For this review, use the dimensioned drawing (mm, ordinates from the lowest corner) and the shaded views. A direction names the side the tool comes from. Give positions to 0.01 mm unless a question says otherwise; leave off trailing zeros. Order: outer loops, then holes, each group sorted by start corner. A loop starts at its lowest first (then second) coordinate and runs counter-clockwise, first axis right, second up.
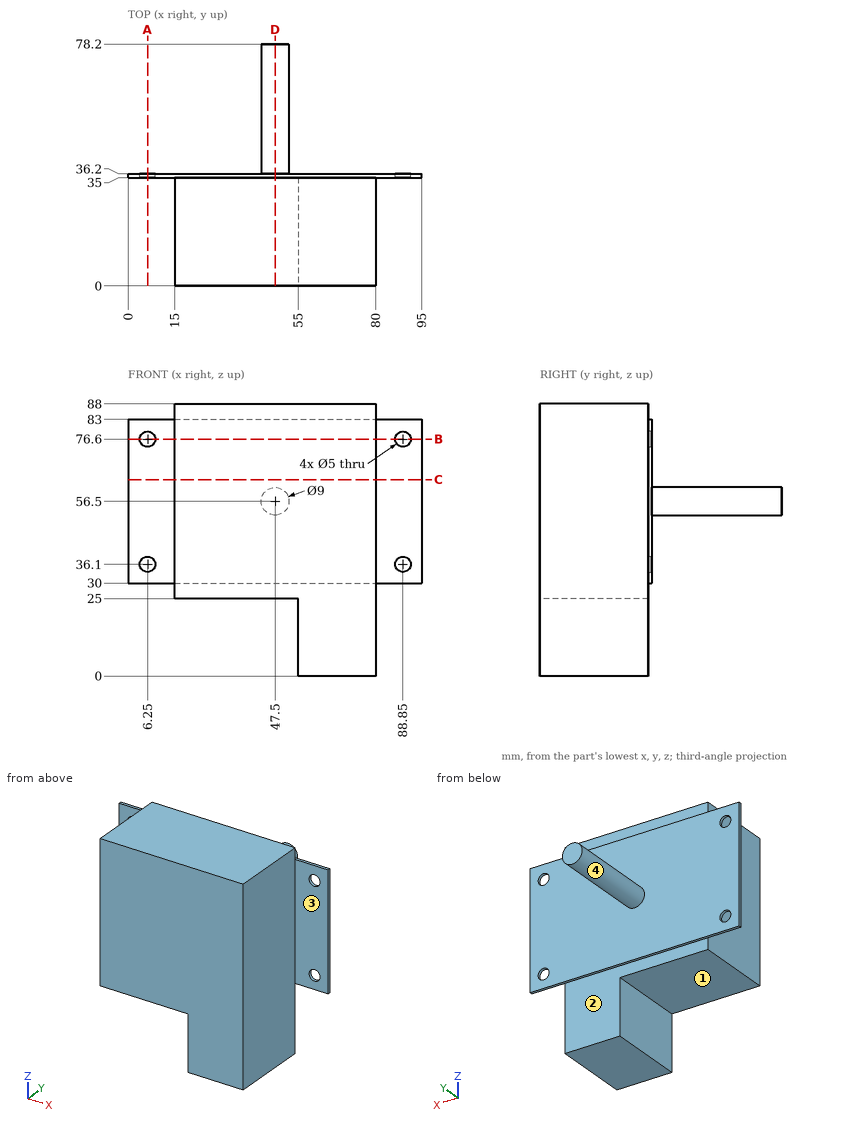
1. For pin 1 (7.5 mm diameter, centred on y = 22.5, z = 18, fed in from -X); pin 2 (10.5 mm diameter, centred on y = 17.5, z = 41, fed in from -X); pin 3 (17.5 mm diameter, centred on y = 25, z = 63, fed in from +X), all flat-tipped, find the tip position at first contact; note any pin that passes through.
Recorded:
pin 1: stops at x = 55
pin 2: stops at x = 15
pin 3: stops at x = 80
2. Take a section at C-C (z = 63.5). State the section outline as (x, y) points, then the cut area to 3 significant figures.
Recorded:
outline: (0, 35) - (15, 35) - (15, 0) - (80, 0) - (80, 35) - (95, 35) - (95, 36.2) - (0, 36.2) - close
area: 2,390 mm2
3. Take a section at A-A (x = 6.25). State the section outline as (y, z) points, then the cut area to 3 significant figures.
Recorded:
outline: (35, 30) - (36.2, 30) - (36.2, 33.6) - (35, 33.6) - close; (35, 38.6) - (36.2, 38.6) - (36.2, 74.1) - (35, 74.1) - close; (35, 79.1) - (36.2, 79.1) - (36.2, 83) - (35, 83) - close
area: 51.6 mm2
4. For line 1 along X through (y, z) = (35.85, 76.6); line 2 along Y through (x, z) = (62.5, 66.5); line 3 along Z through (x, y) = (73, 35.5), list the stretches that pass through material, from the lowest coordinate up.
Recorded:
line 1: x = 0 to 3.75, 8.75 to 86.35, 91.35 to 95
line 2: y = 0 to 36.2
line 3: z = 30 to 83
5. Machinability: for the marked faces 1, 2, 3 and 4, which of the approach directions +Z, -Z, +X, -X, +Y, -Y give a long, thin tool a straight path to every point of the face, cutting with its end or side? Answer none if there is none.
Recorded:
face 1: -Z, -X, +Y, -Y
face 2: -Z, +X, -X, +Y
face 3: +Z, -Z, +X, -Y
face 4: +Y
6. Take a section at D-D (x = 47.5). State the section outline as (y, z) points.
Recorded:
outline: (0, 25) - (35, 25) - (35, 30) - (36.2, 30) - (36.2, 52) - (78.2, 52) - (78.2, 61) - (36.2, 61) - (36.2, 83) - (35, 83) - (35, 88) - (0, 88) - close
7. Take a section at B-B (z = 76.6). State the section outline as (x, y) points, then the cut area to 3 significant figures.
Recorded:
outline: (0, 35) - (3.75, 35) - (3.75, 36.2) - (0, 36.2) - close; (8.75, 35) - (15, 35) - (15, 0) - (80, 0) - (80, 35) - (86.35, 35) - (86.35, 36.2) - (8.75, 36.2) - close; (91.35, 35) - (95, 35) - (95, 36.2) - (91.35, 36.2) - close
area: 2,380 mm2
